Autodesk Inventor part; units mm, degrees
ref_plane "Work Plane1" through (0, 0, 0) normal (1, 0, 0) x (0, 1, 0)
ref_plane "Work Plane2" through (0, 0, 0) normal (0.9510565, 0.309017, 0) x (0, 0, 1)
ref_plane "Work Plane3" through (0, 0, 2.3813) normal (0, 0, -1) x (-1, 0, 0)
sketch "Sketch1" plane through (0, 0, 0) normal (0, 0, 1) x (1, 0, 0)
  circle A0 centre (0, 0) radius 23.9806
  dimension "d0" = 47.9612
extrude "Extrusion1" add sketch "Sketch1" along normal blind 4.7625
sketch "Sketch2" plane through (0, 0, 0) normal (0, 0, -1) x (-1, 0, 0)
  circle A0 centre (0, 0) radius 23.9806
  circle A1 centre (0, 0) radius 20
  dimension "d3" = 40
surface extrude "Pitch Diameter" sketch "Sketch2" against normal through all shown no curves A1
ref_plane "Work Plane1" through (0, 0, 0) normal (1, 0, 0) x (0, 1, 0)
ref_plane "Work Plane2" through (0, 0, 0) normal (0.9510565, 0.309017, 0) x (0, 0, 1)
ref_plane "Work Plane3" through (0, 0, 2.3813) normal (0, 0, -1) x (-1, 0, 0)
spur gear teeth "Spur Gear" teeth 10 pitch diameter 40 tip diameter 47.9612 root diameter 29.9612 face width 4.7625 start plane through (0, 0, 0) normal (0, 0, -1) x (-1, 0, 0)
equation "\"d0\" = da_da"
equation "\"d1\" = da_b"
equation "\"d3\" = da_d"
equation "\"d15\" = da_aw"
equation "\"d19\" = da_aw"
properties part number "PINION" material "Steel"
The listing builds one solid part. Answer for the finished solid, in the listing's coordinates (mm). A direction names the side the tool comes from. Coordinates: 2 decimals unless noted, no trailing zeros. Order: outer loops, then holes, each group sorted by start corner. A loop starts at its lowest first (then second) coordinate and runs counter-clockwise, first axis right, second up.
Q1. Given P1, Ø1, axis at x = -4.5, z = 0.5, coming from the -Y side, flat-ended and moving along its own axis, determine where the tip first touches the part or whether it passes through.
Q2. A cutting plane is placed at C-C, the plane y = -11.5. Write down the section's boundary in (x, z).
Q3. A cutting plane is placed at A-A, the plane y = 16. Write down the section's boundary in (x, z), and give its area (3 significant figures).
Q4. For a pull along X with two mould halves and no side action, classify faces 6 (the face through (-14.117, 19.385, 2.348)), 7 (the face through (14.117, -19.385, 2.348)), 8 (the face through (-17.324, -9.006, 2.348)) as pulls with the +X half, pulls with the -X half, needs draft (parallel to the pull), parting line crosses it, or undercut.
Q5. Which of the six approach directions +Z, -Z, +X, -X, +Y, -Y give full straight-line access (tool end or side, diameter ignored) to faces 1 (the face through (-8.818, 17.562, 2.348)), 2 (the face through (13.919, -13.693, 2.348)), 3 (the face through (12.11, 8.82, 2.35)), 4 (the face through (-8.722, -17.469, 2.348)), 5 (the face through (-19.309, 2.897, 2.348))?
Q6. Consider line 1 (Y direction, x = 13.5, z = 4.05); line 2 (X direction, y = 18.5, z = 3.8); line 3 (Y direction, x = 14.5, z = 3.7). Determine where each line is inside the solid, lowest interval first.
Q7. A cutting plane is placed at D-D, the plane x = 9. Write down the section's boundary in (y, z), and give its area (3 significant figures).
Q8. A cutting plane is placed at B-B, the plane x = 17. Write down the section's boundary in (y, z), and give its area (3 significant figures).
Answers follow:
1. P1: stops at y = -14.44
2. outline: (-12.67, 0) - (12.67, 0) - (12.67, 4.76) - (-12.67, 4.76) - close
3. outline: (-14.9, 0) - (-7.35, 0) - (-7.35, 4.76) - (-14.9, 4.76) - close; (-3.52, 0) - (3.52, 0) - (3.52, 4.76) - (-3.52, 4.76) - close; (7.35, 0) - (14.9, 0) - (14.9, 4.76) - (7.35, 4.76) - close
3. area: 105 mm2
4. face 6: pulls with the -X half
4. face 7: pulls with the +X half
4. face 8: undercut
5. face 1: +Z, -Z, +Y
5. face 2: +Z, -Z, +X
5. face 3: +Z, -Z
5. face 4: +Z, -Z, -Y
5. face 5: +Z, -Z, -X
6. line 1: y = -19.82 to -12.89, -8.09 to 8.09, 12.89 to 19.82
6. line 2: x = -15.26 to -9.85, -3.33 to 3.33, 9.85 to 15.26
6. line 3: y = -19.1 to -14.97, -8.4 to 8.4, 14.97 to 19.1
7. outline: (-17.74, 0) - (17.74, 0) - (17.74, 4.76) - (-17.74, 4.76) - close
7. area: 169 mm2
8. outline: (-8.96, 0) - (-1.85, 0) - (-1.85, 4.76) - (-8.96, 4.76) - close; (1.85, 0) - (8.96, 0) - (8.96, 4.76) - (1.85, 4.76) - close
8. area: 67.7 mm2
